Autodesk Inventor part; units mm, degrees
ref_plane "YZ Plane" through (0, 0, 0) normal (1, 0, 0) x (0, 1, 0)
ref_plane "XZ Plane" through (0, 0, 0) normal (0, 1, 0) x (-1, 0, 0)
ref_plane "XY Plane" through (0, 0, 0) normal (0, 0, 1) x (1, 0, 0)
sketch "Sketch1" plane through (0, 0, 0) normal (0, 1, 0) x (-1, 0, 0)
  line L0 (-8.128, 10.6426) -> (8.128, 10.6426)
  line L1 (8.128, 10.6426) -> (8.128, -10.6426)
  line L2 (8.128, -10.6426) -> (-8.128, -10.6426)
  line L3 (-8.128, -10.6426) -> (-8.128, 10.6426)
  line L4 (-8.128, 10.6426) -> (8.128, -10.6426) construction
  line L5 (8.128, 10.6426) -> (-8.128, -10.6426) construction
  point P0 (0, 0)
  dimension "d0" = 21.2852
  dimension "d1" = 16.256
extrude "Plate1" add sketch "Sketch1" along normal blind 1.524
sketch "Sketch2" plane through (-6.604, 0, 10.6426) normal (-1, 0, 0) x (0, -1, 0)
  line L0 (0, -21.2852) -> (0, 0)
  line L1 (0, 0) -> (-15.5956, 0)
  line L2 (-15.5956, 0) -> (-15.5956, -21.2852)
  line L3 (-15.5956, -21.2852) -> (0, -21.2852)
edge flange "Flange1" height 15.5956 angle 90 thickness 1.524 bend radius 1.524 thickness toward (-1, 0, 0) relief tear relief width 1.524 relief depth 0.762 edges at (-8.128, 1.524, 0) wall of the first edge with corners at (-6.604, 0, -10.6426) (-6.604, 0, 10.6426) (-6.604, 15.5956, 10.6426) (-6.604, 15.5956, -10.6426)
bend "Bend1"
corner "Corner1"
sketch "Sketch3" plane through (-6.604, 15.5956, 10.6426) normal (1, 0, 0) x (0, 0, -1)
  line L0 (0, 0) -> (0, -12.5476) construction
  line L1 (21.2852, -12.5476) -> (21.2852, 0) construction
  circle A0 centre (3.7973, -6.2738) radius 1.5875 construction
  circle A1 centre (17.4879, -6.2738) radius 1.5875 construction
  line L2 (3.7973, -6.2738) -> (17.4879, -6.2738) construction
  line L3 (21.2852, 0) -> (0, 0) construction
  line L4 (10.6426, 0) -> (10.6426, -12.5476) construction
  line L5 (0, -12.5476) -> (21.2852, -12.5476) construction
  line L6 (17.1196, -10.7188) -> (17.8562, -10.7188)
  line L7 (19.4437, -9.1313) -> (19.4437, -3.4163)
  line L8 (17.8562, -1.8288) -> (17.1196, -1.8288)
  line L9 (15.5321, -3.4163) -> (15.5321, -9.1313)
  line L10 (15.5321, -10.7188) -> (19.4437, -1.8288) construction
  line L11 (19.4437, -10.7188) -> (15.5321, -1.8288) construction
  arc A2 (17.1196, -1.8288) -> (15.5321, -3.4163) centre (17.1196, -3.4163) ccw
  arc A3 (19.4437, -3.4163) -> (17.8562, -1.8288) centre (17.8562, -3.4163) ccw
  arc A4 (15.5321, -9.1313) -> (17.1196, -10.7188) centre (17.1196, -9.1313) ccw
  arc A5 (17.8562, -10.7188) -> (19.4437, -9.1313) centre (17.8562, -9.1313) ccw
  line L12 (3.429, -10.7188) -> (4.1656, -10.7188)
  line L13 (5.7531, -9.1313) -> (5.7531, -3.4163)
  line L14 (4.1656, -1.8288) -> (3.429, -1.8288)
  line L15 (1.8415, -3.4163) -> (1.8415, -9.1313)
  line L16 (1.8415, -10.7188) -> (5.7531, -1.8288) construction
  line L17 (5.7531, -10.7188) -> (1.8415, -1.8288) construction
  arc A6 (3.429, -1.8288) -> (1.8415, -3.4163) centre (3.429, -3.4163) ccw
  arc A7 (5.7531, -3.4163) -> (4.1656, -1.8288) centre (4.1656, -3.4163) ccw
  arc A8 (4.1656, -10.7188) -> (5.7531, -9.1313) centre (4.1656, -9.1313) ccw
  arc A9 (1.8415, -9.1313) -> (3.429, -10.7188) centre (3.429, -9.1313) ccw
  point P0 (10.6426, -15.5956)
  point P1 (10.6426, -6.2738)
  dimension "d13" = 13.6906
  dimension "d14" = 3.175
  dimension "d15" = 3.175
  dimension "d16" = 3.9116
  dimension "d17" = 8.89
  dimension "d18" = 1.5875
  dimension "d19" = 3.9116
  dimension "d20" = 8.89
  dimension "d21" = 1.5875
sketch "Sketch4" plane through (0, 1.524, 0) normal (0, 1, 0) x (1, 0, 0)
  line L0 (-5.08, 10.6426) -> (8.128, 10.6426) construction
  line L1 (4.3815, 4.8768) -> (-1.3335, 4.8768) construction
  line L2 (-2.921, 6.4643) -> (-2.921, 7.2009) construction
  line L3 (-1.3335, 8.7884) -> (4.3815, 8.7884) construction
  line L4 (5.969, 7.2009) -> (5.969, 6.4643) construction
  arc A0 (-2.921, 6.4643) -> (-1.3335, 4.8768) centre (-1.3335, 6.4643) ccw construction
  arc A1 (-1.3335, 8.7884) -> (-2.921, 7.2009) centre (-1.3335, 7.2009) ccw construction
  arc A2 (4.3815, 4.8768) -> (5.969, 6.4643) centre (4.3815, 6.4643) ccw construction
  arc A3 (5.969, 7.2009) -> (4.3815, 8.7884) centre (4.3815, 7.2009) ccw construction
  line L5 (8.128, 10.6426) -> (8.128, -10.6426)
  line L6 (1.524, 4.8768) -> (1.524, 8.7884) construction
  line L7 (4.3815, -8.7884) -> (-1.3335, -8.7884)
  line L8 (-2.921, -7.2009) -> (-2.921, -6.4643)
  line L9 (-1.3335, -4.8768) -> (4.3815, -4.8768)
  line L10 (5.969, -6.4643) -> (5.969, -7.2009)
  arc A4 (-2.921, -7.2009) -> (-1.3335, -8.7884) centre (-1.3335, -7.2009) ccw
  arc A5 (-1.3335, -4.8768) -> (-2.921, -6.4643) centre (-1.3335, -6.4643) ccw
  arc A6 (4.3815, -8.7884) -> (5.969, -7.2009) centre (4.3815, -7.2009) ccw
  arc A7 (5.969, -6.4643) -> (4.3815, -4.8768) centre (4.3815, -6.4643) ccw
  line L11 (1.524, -8.7884) -> (1.524, -4.8768) construction
  line L12 (8.128, -10.6426) -> (-5.08, -10.6426) construction
  point P0 (0, 0)
  point P1 (1.524, 6.8326)
  point P2 (1.524, -6.8326)
  dimension "d26" = 1.5875
  dimension "d32" = 3.9116
  dimension "d33" = 8.89
  dimension "d34" = 6.604
  dimension "d35" = 3.81
  dimension "d36" = 1.5875
  dimension "d37" = 3.9116
  dimension "d38" = 8.89
  dimension "d39" = 3.81
  dimension "d40" = 6.604
extrude "Extrusion1" cut sketch "Sketch3" against normal through all
extrude "Extrusion3" cut sketch "Sketch4" against normal through all
equation "\"d3\" = BendReliefWidth"
equation "\"d4\" = BendReliefDepth"
equation "\"d5\" = MinimumRemnant"
equation "\"d6\" = BendRadius"
equation "\"d9\" = BendRadius"
equation "\"d10\" = CornerReliefSize"
equation "\"d11\" = GapSize"
equation "\"d12\" = JacobiRadiusSize"
equation "\"BendRadius\" = Thickness"
equation "\"BendReliefWidth\" = Thickness"
equation "\"BendReliefDepth\" = 0.5 * Thickness"
equation "\"CornerReliefSize\" = 4 * Thickness"
equation "\"MinimumRemnant\" = 2 * Thickness"
equation "\"TransitionRadius\" = BendRadius"
equation "\"JacobiRadiusSize\" = BendRadius"
equation "\"GapSize\" = Thickness"
equation "\"d2\" = BendRadius"
properties part number "mezzanineBracketLeft"
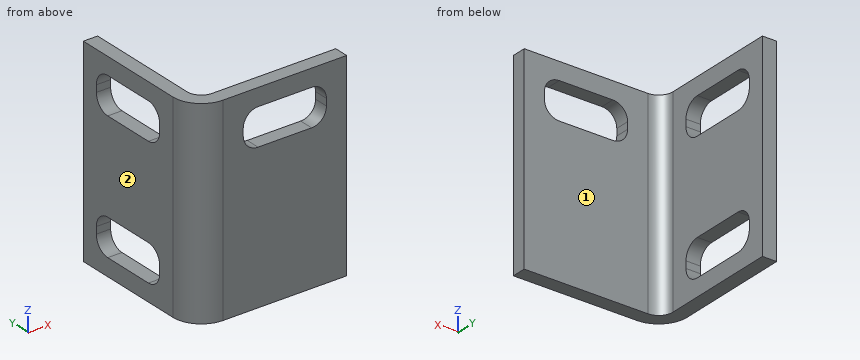
Can you work these out from the model? Positions are in its coordinate system, mm. Face numbers are marked on the shaded views. A direction names the side the tool comes from. Give positions to 0.01 mm unless a question says otherwise; leave off trailing zeros. Order: outer loops, then holes, each group sorted by start corner. A loop starts at its lowest first (then second) coordinate and runs counter-clockwise, first axis right, second up. Notation, with made-up numbers: M -14,28 L 41,28 A20 ccw 41,59 Z; hole C 32,-31 d4. An arc over 180 degrees is marked long. One line per item, written item: value.
1) I want a section at C-C, the plane z = 4.5. List the corners of the cut face in (x, y) for me, plus the area to 3 significant figures.
Answer sheet:
outline: M -8.13,3.05 A3.05 ccw -5.08,0 L 8.13,0 L 8.13,1.52 L -5.08,1.52 A1.52 cw -6.6,3.05 L -6.6,15.6 L -8.13,15.6 Z
area: 44.7 mm^2
2) I want a section at D-D, the plane z = -7.5. List the corners of the cut face in (x, y) for me, plus the area to 3 significant figures.
Answer sheet:
outline: M -8.13,3.05 A3.05 ccw -5.08,0 L 8.13,0 L 8.13,1.52 L -5.08,1.52 A1.52 cw -6.6,3.05 L -6.6,4.9 L -8.13,4.9 Z; M -8.13,13.74 L -6.6,13.74 L -6.6,15.6 L -8.13,15.6 Z
area: 31.3 mm^2
3) I want a section at A-A, the plane x = 2.75. List the corners of the cut face in (y, z) for me, plus the area to 3 significant figures.
Answer sheet:
outline: M 0,-10.64 L 1.52,-10.64 L 1.52,4.88 L 0,4.88 Z; M 0,8.79 L 1.52,8.79 L 1.52,10.64 L 0,10.64 Z
area: 26.5 mm^2
4) Please list where these lines run through material, in increasing order: line 1 along Z through (x, y) = (-7.5, 9.25); line 2 along X through (y, z) = (10, 2.5); line 3 along Y through (x, z) = (-1.5, -2.5).
Answer sheet:
line 1: z = -10.64 to -8.8, -4.89 to 4.89, 8.8 to 10.64
line 2: x = -8.13 to -6.6
line 3: y = 0 to 1.52
5) I want a section at B-B, the plane y = 8. List the corners of the cut face in (x, z) for me, plus the area to 3 significant figures.
Answer sheet:
outline: M -8.13,-10.64 L -6.6,-10.64 L -6.6,-8.8 L -8.13,-8.8 Z; M -8.13,-4.89 L -6.6,-4.89 L -6.6,4.89 L -8.13,4.89 Z; M -8.13,8.8 L -6.6,8.8 L -6.6,10.64 L -8.13,10.64 Z
area: 20.5 mm^2
6) On a 3-axis mill with a long thin cutter (end or side, diameter ignored), from which of +Z, -Z, +X, -X, +Y, -Y can I reach the whole of each face in a straight line? I mean the marked faces 1 and 2. Say none if no direction works.
Answer sheet:
face 1: +Z, -Z, +X, +Y
face 2: +Z, -Z, -X, +Y, -Y
7) For P1, Ø0.6, axis at x = -7.5, z = -7, coming from the -Y side; P2, Ø0.6, axis at x = -7, z = 7, coming from the -Y side; P3, Ø4, axis at y = 12.5, z = -3, coming from the +X side; P4, Ø8, axis at x = 4, z = -8, coming from the -Y side, each with a flat end and sliding along its axis, tell me the tip position at first contact or that it passes through.
Answer sheet:
P1: stops at y = 0.86
P2: stops at y = 0.47
P3: stops at x = -6.6
P4: stops at y = 0
